from build123d import *


with BuildPart() as part:
    # Esquisse1 → Révolution1 (revolve)
    with BuildSketch(Plane.XY, mode=Mode.PRIVATE) as r_volution1_sk:
        with BuildLine():
            Line((2, 6.5), (3, 6.5))
            Line((3, 6.5), (3, 3))
            Line((3, 3), (3.5, 3))
            Line((3.5, 3), (3.5, 2))
            Line((3.5, 2), (-3, 2))
            Line((-3, 2), (-3, 6.5))
            Line((-3, 6.5), (-2, 6.5))
            ThreePointArc((-2, 6.5), (0, 5.5), (2, 6.5))
        make_face()
    revolve(r_volution1_sk.sketch.rotate(Axis((0, 0, 0), (1, 0, 0)), 90), axis=Axis((0, 0, 0), (1, 0, 0)))


solid = part.part
The model under review builds one solid part; all positions refer to its coordinate system, in mm. A direction names the side the tool comes from. Coordinates: 2 decimals unless noted, no trailing zeros. Order: outer loops, then holes, each group sorted by start corner. A loop starts at its lowest first (then second) coordinate and runs counter-clockwise, first axis right, second up. Notation, with made-up numbers: (5.25, -36.5) -> (33.25, -36.5) arc R11 ccw to (33.25, -16.5) -> close; hole circle Ø2 at (-31, 80). An arc over 180 degrees is marked (long way). Answer in a Markdown table with one row per item.
(1) Consider section C-C (x = -1.5). Write out the cut boundary in (y, z), plus the area to 3 significant figures.
Answers:
| item | result |
|---|---|
| outline | circle Ø12 at (0, 0); hole circle Ø4 at (0, 0) |
| area | 101 mm² |
(2) Wall thickness on line 1 along X through (y, z) = (3.75, -4.5); line 2 along Z through (x, y) = (-2.5, -1.75); line 3 along Y through (x, z) = (1, 0): over which ranges is each line inside the solid? List them lowest first.
Answers:
| item | result |
|---|---|
| line 1 | -3 to -1.29, 1.29 to 3 |
| line 2 | -6.26 to -0.97, 0.97 to 6.26 |
| line 3 | -5.71 to -2, 2 to 5.71 |
(3) Machinability: for faces 4 (the cylindrical face through (3.25, -0.9, 2.86)), 5 (the cylindrical face through (-2.493, 3.955, -5.158)), which of the approach directions +Z, -Z, +X, -X, +Y, -Y give a long, thin tool a straight path to every point of the face, cutting with its end or side? Answer none if there is none.
Answers:
| item | result |
|---|---|
| face 4 | +X |
| face 5 | +X, -X |
(4) Consider section A-A (z = 0). Write out the cut boundary in (x, y), plus the area to 3 significant figures.
Answers:
| item | result |
|---|---|
| outline | (-3, -6.5) -> (-2, -6.5) arc R2.5 cw to (2, -6.5) -> (3, -6.5) -> (3, -3) -> (3.5, -3) -> (3.5, -2) -> (-3, -2) -> close; (-3, 2) -> (3.5, 2) -> (3.5, 3) -> (3, 3) -> (3, 6.5) -> (2, 6.5) arc R2.5 cw to (-2, 6.5) -> (-3, 6.5) -> close |
| area | 49.4 mm² |
(5) The part is to be moulded in two halves that separate along Y. For faces 1 (the cylindrical face through (0, 2, 0)), 2 (the flat face through (-3, -2, -1)), 3 (the cylindrical face through (2.507, 3.955, -5.158)), say which applies: +Y half, -Y half, draft (parallel to the pull), parting line (faces both ways), or undercut.
Answers:
| item | result |
|---|---|
| face 1 | undercut |
| face 2 | draft |
| face 3 | parting line |
(6) Consider section D-D (x = 0.25). Write out the cut boundary in (y, z), plus the area to 3 significant figures.
Answers:
| item | result |
|---|---|
| outline | circle Ø11.03 at (0, 0); hole circle Ø4 at (0, 0) |
| area | 82.9 mm² |
(7) Insertion check: pin 1 (1.5 mm diameter, centred on x = 1.5, z = 3, fed in from -Y); pin 2 (2 mm diameter, centred on y = -1.5, z = 4.5, fed in from +X). Each pin has a flat end and moves straight along its axis. Give the tip position at first contact, or say it passes through.
Answers:
| item | result |
|---|---|
| pin 1 | y = -6.02 |
| pin 2 | x = 3 |
